Design review of the part built by this model. Coordinates are the model's own, in mm. A direction names the side the tool comes from. Give positions to 0.01 mm unless a question says otherwise; leave off trailing zeros. Loops run counter-clockwise (first coordinate to the right, second up) from the corner with the lowest first, then second, coordinate; pieces in that order, holes last. Notation, with made-up numbers: M 72,88.5 L 79,88.5 A34 ccw 79,124.5 Z; hole C 40,36.5 d6. An arc over 180 degrees is marked long. Answer as CSV lines item,"result".
Autodesk Inventor part; units mm, degrees
ref_plane "YZ Plane" through (0, 0, 0) normal (1, 0, 0) x (0, 1, 0)
ref_plane "XZ Plane" through (0, 0, 0) normal (0, 1, 0) x (-1, 0, 0)
ref_plane "XY Plane" through (0, 0, 0) normal (0, 0, 1) x (1, 0, 0)
sketch "Skizze1" plane through (0, 0, 0) normal (1, 0, 0) x (0, 1, 0)
  line L0 (0, 18.5) -> (-6, 18.5)
  line L1 (-6, 18.5) -> (-6, 5.5)
  line L2 (-24, 0) -> (0, 0)
  line L3 (0, 0) -> (0, 18.5)
  line L4 (-24, 0) -> (-24, 5.5)
  line L5 (-24, 5.5) -> (-6, 5.5)
  dimension "d0" = 18.5
  dimension "d1" = 6
  dimension "d2" = 5.5
  dimension "d3" = 24
extrude "Extrusion1" add sketch "Skizze1" along normal mid plane 25
sketch "Skizze2" plane through (-12.5, 0, 18.5) normal (0, 1, 0) x (1, 0, 0)
  line L0 (25, 18.5) -> (25, 0)
  line L1 (25, 18.5) -> (0, 18.5)
  line L2 (0, 0) -> (0, 18.5)
  line L3 (0, 0) -> (25, 0) construction
  line L4 (12.5, 0) -> (12.5, 18.5) construction
  line L5 (0, 0) -> (25, 0)
  point P0 (12.5, 4.5)
hole "Bohrung1" at (0, 0, 14) direction (0, -1, 0) diameter 4.917 end through all
chamfer "Fase1" [suppressed]
fillet "Rundung1" radius 0.5 2 edges at (12.5, -6, 12) (-12.5, -6, 12)
fillet "Rundung2" [suppressed]
sketch "Skizze5" plane through (-12.5, 0, 18.5) normal (0, 1, 0) x (1, 0, 0)
  line L0 (25, 18.5) -> (0, 18.5)
  line L1 (0, 0) -> (0, 18.5)
  line L2 (25, 18.5) -> (0, 18.5)
  line L3 (0, 18.5) -> (0, 13)
  line L4 (0, 13) -> (25, 13)
  line L5 (25, 13) -> (25, 18.5)
  line L6 (25, 13) -> (25, 18.5)
  line L7 (0, 18.5) -> (0, 13)
  line L8 (0, 18.5) -> (25, 18.5)
  line L9 (0, 13) -> (25, 13)
  point P0 (12.5, 18.5)
  point P1 (1, 16.5)
  point P2 (24, 16.5)
sketch "Sketch7" plane through (-12.5, -8, 5.5) normal (0, 0, 1) x (1, 0, 0)
  line L0 (25, 8) -> (0, 8)
  line L1 (-14.5, -26) -> (39.5, -26) construction
  line L2 (39.5, -26) -> (39.5, -16)
  line L3 (39.5, -16) -> (-14.5, -16)
  line L4 (-14.5, -16) -> (-14.5, -26)
  line L5 (10.0415, 8) -> (14.9585, 8) construction
  line L6 (12.5, 8) -> (12.5, -16) construction
  arc A0 (39.5, -26) -> (-14.5, -26) centre (12.5, -274.5377) ccw
  dimension "d44" = 54
  dimension "d45" = 10
  dimension "d46" = 24
  dimension "d47" = 250
extrude "Extrusion2" add sketch "Sketch7" against normal up to surface (5.5 mm away) from surface at 0
fillet "Fillet3" radius 2 2 edges at (27, -34, 2.75) (-27, -34, 2.75)
fillet "Fillet3" radius 4 4 edges at (12.5, -24, 2.75) (-12.5, -24, 2.75) (27, -24, 2.75) (-27, -24, 2.75)
fillet "Fillet4" radius 3 1 edges at (0, -6, 5.5)
equation "\"d46\" = d3"
properties part number "Chip Kick Vorne" material "Steel, Carbon"
1. For P1, Ø1.6, axis at x = 21.5, z = 2.5, coming from the +Y side; P2, Ø3, axis at x = 12.5, z = 15, coming from the -Y side; P3, Ø7.5, axis at x = -3.5, y = -22, coming from the +Z side; P4, Ø10, axis at y = -20.5, z = 11, coming from the -X side, all flat-tipped, find the tip position at first contact; note any pin that passes through.
Answer block:
P1,"y = -24"
P2,"y = -6"
P3,"z = 5.5"
P4,"through"
2. We need section B-B, the plane x = 0. Write out the cut boundary in (y, z).
Answer block:
outline,"M -32.54,0 L 0,0 L 0,11.54 L -6,11.54 L -6,8.5 A3 cw -9,5.5 L -32.54,5.5 Z; M -6,16.46 L 0,16.46 L 0,18.5 L -6,18.5 Z"
3. The part is to be moulded in two halves that separate along X. For faces 4 (the flat face through (27, -30, 3)), 5 (the flat face through (0, -20, 0)), 6 (the cylindrical face through (-0.108, -3.042, 11.544)), say which applies: pulls with the +X half, pulls with the -X half, needs draft (parallel to the pull), parting line crosses it, or undercut.
Answer block:
face 4,"pulls with the +X half"
face 5,"needs draft"
face 6,"undercut"
4. To check wall thickness, follow L1, parallel to X at y = -4, z = 14; L2, parallel to Z at x = 0, y = -4.3; L3, parallel to Z at x = 2, y = -16. State the ranges of each line that lie inside material, in increasing order. Write a range as [from, to].
Answer block:
L1,"[-12.5, -2.46], [2.46, 12.5]"
L2,"[0, 11.54], [16.46, 18.5]"
L3,"[0, 5.5]"
5. We need section C-C, the plane z = 4. Write out the cut boundary in (x, y), plus the area to 3 significant figures.
Answer block:
outline,"M -27,-31.78 A2 ccw -24.8,-33.77 A250 cw 24.8,-33.77 A2 ccw 27,-31.78 L 27,-28 A4 ccw 23,-24 L 16.5,-24 A4 cw 12.5,-20 L 12.5,0 L -12.5,0 L -12.5,-20 A4 cw -16.5,-24 L -23,-24 A4 ccw -27,-28 Z"
area,"1,090 mm²"
6. We need section A-A, the plane z = 14. Write out the cut boundary in (x, y).
Answer block:
outline,"M -12.5,-5.5 A0.5 ccw -12,-6 L -2.46,-6 L -2.46,0 L -12.5,0 Z; M 2.46,-6 L 12,-6 A0.5 ccw 12.5,-5.5 L 12.5,0 L 2.46,0 Z"
7. We need section D-D, the plane y = -15. Write out the cut boundary in (x, z), plus the area to 4 significant figures.
Answer block:
outline,"M -12.5,0 L 12.5,0 L 12.5,5.5 L -12.5,5.5 Z"
area,"137.5 mm²"
8. For faces 1 (the flat face through (0, -24, 5.5)), 2 (the flat face through (12.5, -8, 5)), 3 (the flat face through (-12.5, -8, 5)), list the 3-axis set-ups (+Z, -Z, +X, -X, +Y, -Y) from which the entire face can be reached by the end or side of a thin tool; tool diameter is ignored.
Answer block:
face 1,"+Z, +X, -X, -Y"
face 2,"+Z, -Z, +X, +Y"
face 3,"+Z, -Z, -X, +Y"
